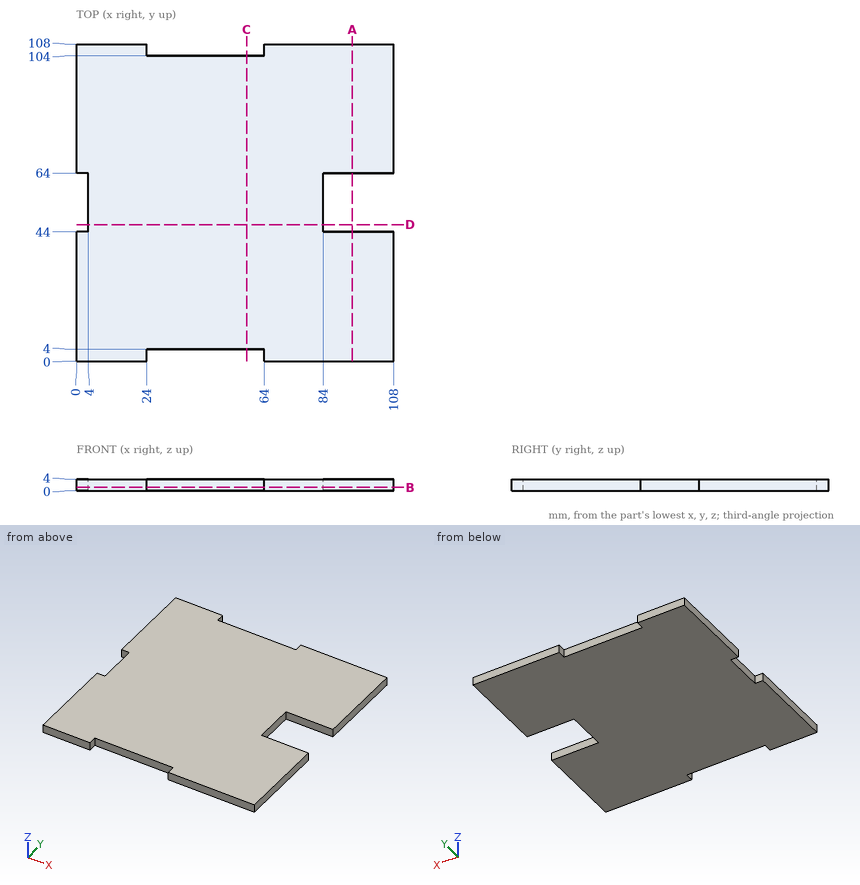
Could you check a few things on this drawing? It's one solid part, dimensions in mm from its lowest x, y, z. Give positions to 0.01 mm unless a question says otherwise; leave off trailing zeros. Write each loop counter-clockwise with the first axis right and the second up, starting at its lowest first coordinate (ties: lowest second). Pieces come first, ordered by that corner, then holes.
(1) Imagine slicing it at D-D, the plane y = 46.5. Write out the boundary of the cut face in (x, z), and give its area (3 significant figures).
Output values:
outline: (4, 0) - (84, 0) - (84, 4) - (4, 4) - close
area: 320 mm2
(2) If I drill on L1, parallel to Y at x = 45, z = 3.65; L2, parallel to X at y = 58, z = 2.25, over which ranges is the centre line in solid material (lowest first)?
Output values:
L1: y = 4 to 104
L2: x = 4 to 84
(3) Imagine slicing it at C-C, the plane x = 58. Write out the boundary of the cut face in (y, z).
Output values:
outline: (4, 0) - (104, 0) - (104, 4) - (4, 4) - close
(4) Will these pins go through, and if not, where does the flat tip stop? pin 1 (1.5 mm diameter, centred on y = 50.5, z = 2, fed in from +X); pin 2 (2 mm diameter, centred on x = 93.5, z = 1, fed in from -Y); pin 3 (2 mm diameter, centred on y = 56.5, z = 3, fed in from -X); pin 4 (1.2 mm diameter, centred on x = 40, z = 1.5, fed in from +Y).
Output values:
pin 1: stops at x = 84
pin 2: stops at y = 0
pin 3: stops at x = 4
pin 4: stops at y = 104
(5) Imagine slicing it at B-B, the plane z = 1.15. Write out the boundary of the cut face in (x, y).
Output values:
outline: (0, 0) - (24, 0) - (24, 4) - (64, 4) - (64, 0) - (108, 0) - (108, 44) - (84, 44) - (84, 64) - (108, 64) - (108, 108) - (64, 108) - (64, 104) - (24, 104) - (24, 108) - (0, 108) - (0, 64) - (4, 64) - (4, 44) - (0, 44) - close
(6) Imagine slicing it at A-A, the plane x = 94. Write out the boundary of the cut face in (y, z).
Output values:
outline: (0, 0) - (44, 0) - (44, 4) - (0, 4) - close; (64, 0) - (108, 0) - (108, 4) - (64, 4) - close
